from build123d import *

# Parameters (mm, degrees)
SKETCH_1_W          = 10
SKETCH_1_H          = 5
EXTRUDE_1_DEPTH     = 0.5
SKETCH_2_W          = 3
SKETCH_2_H          = 3
EXTRUDE_2_DEPTH     = 0.5
SKETCH_3_W          = 10
SKETCH_3_H          = 5
EXTRUDE_3_DEPTH     = 0.5
EXTRUDE_4_DEPTH     = 5
CUT_EXTRUDE_3_DEPTH = 5
SKETCH_6_W          = 1.6
SKETCH_6_H          = 1.6
CUT_EXTRUDE_4_DEPTH = 2.5
SKETCH_7_W          = 10
SKETCH_7_H          = 0.5
CUT_EXTRUDE_5_DEPTH = 1
SKETCH_8_W          = 10
SKETCH_8_H          = 4
EXTRUDE_5_DEPTH     = 1
SKETCH_11_W         = 10
SKETCH_11_H         = 4
SKETCH_11_W_2       = 3
SKETCH_11_H_2       = 3
CUT_EXTRUDE_6_DEPTH = 0.7
CUT_EXTRUDE_7_REACH = 8.595
SKETCH_6_2_W        = 1.6
SKETCH_6_2_H        = 1.6


with BuildPart() as part:
    # 草图1 → 凸台-拉伸1 (new body)
    with BuildSketch(Plane(origin=(0, 0, 0), x_dir=(1, 0, 0), z_dir=(0, 1, 0))):
        Rectangle(SKETCH_1_W, SKETCH_1_H)
    extrude(amount=EXTRUDE_1_DEPTH)

    # 草图2 → 凸台-拉伸2 (add)
    with BuildSketch(Plane(origin=(0, 0.5, 0), x_dir=(1, 0, 0), z_dir=(0, 1, 0))):
        Rectangle(SKETCH_2_W, SKETCH_2_H)
    extrude(amount=EXTRUDE_2_DEPTH)

    # 草图3 → 凸台-拉伸3 (add)
    with BuildSketch(Plane(origin=(0, 1, 0), x_dir=(1, 0, 0), z_dir=(0, 1, 0))):
        Rectangle(SKETCH_3_W, SKETCH_3_H)
    extrude(amount=EXTRUDE_3_DEPTH)

    # 草图4 → 凸台-拉伸4 (add)
    with BuildSketch(Plane.XY.offset(2.5)):
        with BuildLine():
            Line((-5, 1.5), (5, 1.5))
            ThreePointArc((5, 1.5), (0, 3.5), (-5, 1.5))
        make_face()
    extrude(amount=-EXTRUDE_4_DEPTH)

    # 草图5 → 切除-拉伸3 (cut)
    with BuildSketch(Plane.XY.offset(2.5)):
        with BuildLine():
            Line((-4.75, 3.826153858), (-4.25, 3.826153858))
            Line((-4.25, 3.826153858), (-4.25, 1.873670062))
            ThreePointArc((-4.25, 1.873670062), (-4.504363668, 1.680951324), (-4.75, 1.477225575))
            Line((-4.75, 1.477225575), (-4.75, 3.826153858))
        make_face()
        with BuildLine():
            Line((-3.75, 3.826153858), (-3.75, 2.204836823))
            ThreePointArc((-3.75, 2.204836823), (-3.502717622, 2.347713704), (-3.25, 2.480740698))
            Line((-3.25, 2.480740698), (-3.25, 3.826153858))
            Line((-3.25, 3.826153858), (-3.75, 3.826153858))
        make_face()
        with BuildLine():
            Line((-2.75, 3.826153858), (-2.75, 2.708203932))
            ThreePointArc((-2.75, 2.708203932), (-2.501688927, 2.804708114), (-2.25, 2.892024376))
            Line((-2.25, 2.892024376), (-2.25, 3.826153858))
            Line((-2.25, 3.826153858), (-2.75, 3.826153858))
        make_face()
        with BuildLine():
            Line((-1.75, 3.826153858), (-1.75, 3.03562364))
            ThreePointArc((-1.75, 3.03562364), (-1.500932598, 3.092933197), (-1.25, 3.141428429))
            Line((-1.25, 3.141428429), (-1.25, 3.826153858))
            Line((-1.25, 3.826153858), (-1.75, 3.826153858))
        make_face()
        with BuildLine():
            Line((-0.75, 3.826153858), (-0.75, 3.211102551))
            ThreePointArc((-0.75, 3.211102551), (-0.500298955, 3.232717398), (-0.25, 3.245688373))
            Line((-0.25, 3.245688373), (-0.25, 3.826153858))
            Line((-0.25, 3.826153858), (-0.75, 3.826153858))
        make_face()
        with BuildLine():
            Line((0.25, 3.826153858), (0.25, 3.245688373))
            ThreePointArc((0.25, 3.245688373), (0.500298955, 3.232717398), (0.75, 3.211102551))
            Line((0.75, 3.211102551), (0.75, 3.826153858))
            Line((0.75, 3.826153858), (0.25, 3.826153858))
        make_face()
        with BuildLine():
            Line((1.25, 3.826153858), (1.25, 3.141428429))
            ThreePointArc((1.25, 3.141428429), (1.500932598, 3.092933197), (1.75, 3.03562364))
            Line((1.75, 3.03562364), (1.75, 3.826153858))
            Line((1.75, 3.826153858), (1.25, 3.826153858))
        make_face()
        with BuildLine():
            Line((2.25, 3.826153858), (2.25, 2.892024376))
            ThreePointArc((2.25, 2.892024376), (2.501688927, 2.804708114), (2.75, 2.708203932))
            Line((2.75, 2.708203932), (2.75, 3.826153858))
            Line((2.75, 3.826153858), (2.25, 3.826153858))
        make_face()
        with BuildLine():
            Line((3.25, 3.826153858), (3.25, 2.480740698))
            ThreePointArc((3.25, 2.480740698), (3.502717622, 2.347713704), (3.75, 2.204836823))
            Line((3.75, 2.204836823), (3.75, 3.826153858))
            Line((3.75, 3.826153858), (3.25, 3.826153858))
        make_face()
        with BuildLine():
            Line((4.25, 3.826153858), (4.25, 1.873670062))
            ThreePointArc((4.25, 1.873670062), (4.504363668, 1.680951324), (4.75, 1.477225575))
            Line((4.75, 1.477225575), (4.75, 3.826153858))
            Line((4.75, 3.826153858), (4.25, 3.826153858))
        make_face()
    extrude(amount=-CUT_EXTRUDE_3_DEPTH, mode=Mode.SUBTRACT)

    # 草图6 → 切除-拉伸4 (cut)
    with BuildSketch(Plane.XZ):
        Rectangle(SKETCH_6_W, SKETCH_6_H)
    extrude(amount=-CUT_EXTRUDE_4_DEPTH, mode=Mode.SUBTRACT)

    # 草图7 → 切除-拉伸5 (cut)
    with BuildSketch(Plane.XZ):
        with Locations((0, 2.25)):
            Rectangle(SKETCH_7_W, SKETCH_7_H)
        with Locations((0, -2.25)):
            Rectangle(SKETCH_7_W, SKETCH_7_H)
    extrude(amount=-CUT_EXTRUDE_5_DEPTH, mode=Mode.SUBTRACT)

    # 草图8 → 凸台-拉伸5 (add)
    with BuildSketch(Plane.XZ):
        Rectangle(SKETCH_8_W, SKETCH_8_H)
    extrude(amount=EXTRUDE_5_DEPTH)

    # 草图11 → 切除-拉伸6 (cut)
    with BuildSketch(Plane(origin=(0, 0.5, 0), x_dir=(1, 0, 0), z_dir=(0, 1, 0))):
        Rectangle(SKETCH_11_W, SKETCH_11_H)
        Rectangle(SKETCH_11_W_2, SKETCH_11_H_2, mode=Mode.SUBTRACT)
    extrude(amount=-CUT_EXTRUDE_6_DEPTH, mode=Mode.SUBTRACT)

    # 草图6<2> → 切除-拉伸7 (cut, up to next)
    with BuildSketch(Plane.XZ, mode=Mode.PRIVATE) as cut_extrude_7_sk1:
        Rectangle(SKETCH_6_2_W, SKETCH_6_2_H)
    cut_extrude_7_tool1 = extrude(cut_extrude_7_sk1.sketch, amount=CUT_EXTRUDE_7_REACH, mode=Mode.PRIVATE) & part.part
    add(cut_extrude_7_tool1.solids().sort_by_distance((0, 0, 0))[0], mode=Mode.SUBTRACT)


solid = part.part
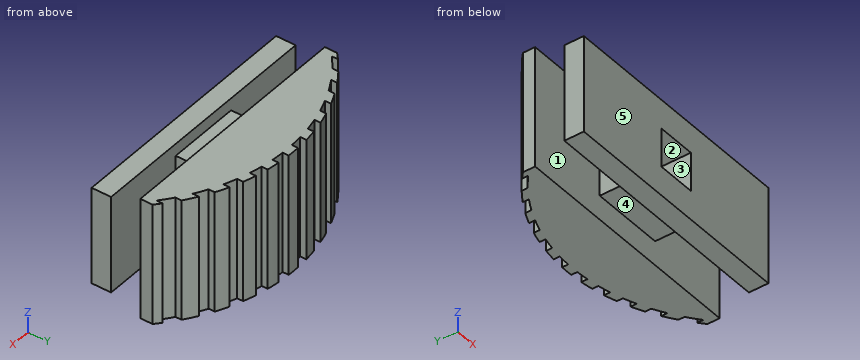
Geometry check sheet. Reference: the model listing, model coordinates, mm. Face numbers are marked on the shaded views. A direction names the side the tool comes from. Give positions to 0.01 mm unless a question says otherwise; leave off trailing zeros. Loops run counter-clockwise (first coordinate to the right, second up) from the corner with the lowest first, then second, coordinate; pieces in that order, holes last. Notation, with made-up numbers: (54, 6.25) -> (98, 6.25) arc R16 ccw to (98, 37.25) -> close; hole circle Ø4 at (35.25, 36.5). An arc over 180 degrees is marked (long way). Answer in a Markdown table with one row per item. Add a question column.
1) Gauge pin test, flat ends, axial feed: P1, Ø0.6, axis at x = -0.5, y = 0.5, coming from the -Z side; P2, Ø0.8, axis at y = 0.5, z = 0.5, coming from the -X side; P3, Ø0.6, axis at x = 1, y = -0.5, coming from the +Z side. Record the tip position at first contact, or that the pin passes through.
2) Cross-section at C-C on y = 0.6. Record the boundary of the cut face in (x, z), and give its area (3 significant figures).
3) Cross-section at A-A on x = 3.5. Record the boundary of the cut face in (y, z).
4) Draft check along X on the marked faces 1 and 2. Enter one of: pulls with the +X half, pulls with the -X half, needs draft (parallel to the pull), parting line crosses it, or undercut.
5) Material ranges on probe 1 along Z at (x, y) = (0.25, -0.05); probe 2 along Y at (x, z) = (0, -1.8), recorded low to high. Write a range as from..to.
6) Set-up check for the marked faces 3, 4 and 5: record each of +Z, -Z, +X, -X, +Y, -Y from which the full face is reachable in a straight line by a thin tool's end or side.
7) Cross-section at D-D on x = 2. Record the boundary of the cut face in (y, z), and give its area (3 significant figures).
8) Cross-section at B-B on y = -0.6. Record the boundary of the cut face in (x, z).
Outcome:
| question | item | result |
|---|---|---|
| 1 | P1 | stops at z = -1.5 |
| 1 | P2 | stops at x = -1.5 |
| 1 | P3 | stops at z = 2 |
| 2 | outline | (-1.5, -1.5) -> (1.5, -1.5) -> (1.5, 1.5) -> (-1.5, 1.5) -> close; hole (-0.8, -0.8) -> (0.8, -0.8) -> (0.8, 0.8) -> (-0.8, 0.8) -> close |
| 2 | area | 6.44 mm^2 |
| 3 | outline | (-1, -2) -> (-0.2, -2) -> (-0.2, 2) -> (-1, 2) -> close; (1, -2.5) -> (2.35, -2.5) -> (2.35, 2.5) -> (1, 2.5) -> close |
| 4 | face 1 | needs draft |
| 4 | face 2 | undercut |
| 5 | probe 1 | z = -1.5..-0.8, 0.8..1.5 |
| 5 | probe 2 | y = -1..-0.2, 1..3.5 |
| 6 | face 3 | -Y |
| 6 | face 4 | -Z, +X, -X |
| 6 | face 5 | +Z, -Z, +X, -X, -Y |
| 7 | outline | (-1, -2) -> (-0.2, -2) -> (-0.2, 2) -> (-1, 2) -> close; (1, -2.5) -> (3.22, -2.5) -> (3.22, 2.5) -> (1, 2.5) -> close |
| 7 | area | 14.3 mm^2 |
| 8 | outline | (-5, -2) -> (5, -2) -> (5, 2) -> (-5, 2) -> close; hole (-0.8, -0.8) -> (0.8, -0.8) -> (0.8, 0.8) -> (-0.8, 0.8) -> close |
